Part model, mm, in its own coordinate system. A direction names the side the tool comes from. Coordinates: 2 decimals unless noted, no trailing zeros. Use a Markdown table: item, result. Add a question column.
Q1. Mould opens along Y. For faces 1 (the flat face through (-19.05, -601, 137)), 2 (the flat face through (-515, -1200.15, 79)), 3 (the flat face through (-521, -1219.2, 87)), 4 (the flat face through (0, -601, 150)) say: released by +Y, released by -Y, zero draft, split by the parting line, or undercut.
Q2. Tool access for faces 5 (the flat face through (-1804, -601, 19.05)), 6 (the flat face through (-521, 0, 87)), 7 (the flat face through (-515, -19.05, 79)): list every direction of +Z, -Z, +X, -X, +Y, -Y with a clear straight run to the whole face (end or side of a thin tool).
Q3. Wall check: L1, parallel to Y at x = -82.5, z = 126.5; L2, parallel to Z at x = -714, y = -730; L3, parallel to Z at x = -513, y = -835.5. Give the ranges that are in metal, low to high. Write a range as from..to.
Q4. Pin check, flat tips, straight feed: pin 1 Ø5.5 at (y, z) = (-392, 6) entering from -X; pin 2 Ø8 at (x, z) = (-735.5, 61.5) entering from +Y; pin 3 Ø1 at (x, y) = (-548.5, -654) entering from +Z; pin 4 Ø3 at (x, y) = (-844.5, -389.5) entering from -Z. Stop position of each tip, or through.
from build123d import *

# Parameters (mm, degrees)
F1_DEPTH = 1219.2
F2_T     = -19.05


with BuildPart() as f1:
    # F0 (on Front) → F1 (new body)
    with BuildSketch(Plane.XZ):
        with BuildLine():
            Line((-1778, 0), (0, 0))
            Line((0, 0), (0, 304.8))
            add(Edge.make_bspline(
                [(0, 304.8), (-762.4312639236, 30.0072385311), (-1787.0007753372, 39.029404521), (-1828.8, 38.1)],
                knots=[0, 0, 0, 0, 1848.1445641508, 1848.1445641508, 1848.1445641508, 1848.1445641508], degree=3))
            Line((-1828.8, 38.1), (-1828.8, 19.05))
            Line((-1828.8, 19.05), (-1778, 19.05))
            Line((-1778, 19.05), (-1778, 0))
        make_face()
    extrude(amount=F1_DEPTH)

    # F2
    f2_openings = [f1.faces().sort_by_distance(p)[0] for p in [
        (-889, -609.6, 0),
    ]]
    offset(amount=F2_T, openings=f2_openings, kind=Kind.INTERSECTION)


solid = f1.part
Recorded:
| question | item | result |
|---|---|---|
| 1 | face 1 | undercut |
| 1 | face 2 | undercut |
| 1 | face 3 | released by -Y |
| 1 | face 4 | zero draft |
| 2 | face 5 | -Z, -X, +Y, -Y |
| 2 | face 6 | +Z, -Z, +X, -X, +Y |
| 2 | face 7 | -Z |
| 3 | L1 | -1219.2..-1200.15, -19.05..0 |
| 3 | L2 | 108.41..127.71 |
| 3 | L3 | 145.12..164.56 |
| 4 | pin 1 | x = -1778 |
| 4 | pin 2 | y = 0 |
| 4 | pin 3 | z = 157.55 |
| 4 | pin 4 | z = 88.39 |
